The listing builds one solid part. Answer for the finished solid, in the listing's coordinates (mm). A direction names the side the tool comes from. Round coordinates to 2 decimals unless told otherwise and drop trailing zeros. Write each loop counter-clockwise with the first axis right and the second up, starting at its lowest first coordinate (ties: lowest second). Pieces come first, ordered by that corner, then holes. Notation, with made-up numbers: (31, 29) - (49, 29) arc R23 cw to (49, 66) - close; hole circle Ø8 at (25, 39). An arc over 180 degrees is marked (long way). Answer as CSV lines item,"result". Start each with the question number.
Item 1: A cutting plane is placed at A-A on y = -20.5. Determine the outline of the cut face in (x, z).
Item 2: Which of the six approach directions +Z, -Z, +X, -X, +Y, -Y give full straight-line access (tool end or side, diameter ignored) to faces 4 (the flat face through (5.197, 21, -1)), 5 (the flat face through (-21.197, -41, -1)), 6 (the flat face through (-21.197, 21, -1)), 7 (the flat face through (-13, -30.6, -1))?
Item 3: A cutting plane is placed at B-B on y = 14.65. Determine the outline of the cut face in (x, z), and give its area (3 significant figures).
Item 4: For a pull along Y with two mould halves and no side action, classify faces 1 (the flat face through (2.697, -10, -1)), 2 (the flat face through (5.197, -41, -1)), 3 (the flat face through (24, -40.1, -1)) as pulls with the +Y half, pulls with the -Y half, needs draft (parallel to the pull), parting line crosses it, or undercut.
Item 5: A flat-ended cylindrical pin translates along its axis: pin 1 (0.8 mm diameter, centred on y = -41.5, z = -1.5, fed in from +X). Find the tip coordinate at first contact, or state that the pin passes through.
Item 6: Straight lines are drawn through the part: line 1 along X through (y, z) = (-18, -0.75); line 2 along Y through (x, z) = (8, -0.4); line 3 along Y through (x, z) = (-12, -0.6). For each, find the intervals that lie inside material, in ascending order. Write a range as [from, to].
Item 7: A cutting plane is placed at D-D on z = -1.25. State how many separate pieces and enclosed holes the cut face has, and give its area (3 significant figures).
Item 8: A cutting plane is placed at C-C on x = -4. Determine the outline of the cut face in (y, z).
```python
from build123d import *

# Parameters (mm, degrees)
SKETCH_1_W      = 54
SKETCH_1_H      = 60
SKETCH_1_R      = 1.75
SKETCH_1_W_2    = 21
SKETCH_1_H_2    = 41
SKETCH_1_W_3    = 16
SKETCH_1_H_3    = 2.5
EXTRUDE_1_DEPTH = 3


with BuildPart() as part:
    # Эскиз1 → Бобышка-Вытянуть1 (new body)
    with BuildSketch(Plane.XY):
        with Locations((0, -10.1)):
            Rectangle(SKETCH_1_W, SKETCH_1_H)
        with Locations((-18.19729, 14.65)):
            Circle(SKETCH_1_R, mode=Mode.SUBTRACT)
        with Locations((-8.19729, 14.65)):
            Circle(SKETCH_1_R, mode=Mode.SUBTRACT)
        with Locations((8.19729, 14.65)):
            Circle(SKETCH_1_R, mode=Mode.SUBTRACT)
        with Locations((18.19729, 14.65)):
            Circle(SKETCH_1_R, mode=Mode.SUBTRACT)
        with Locations((18.19729, -34.85)):
            Circle(SKETCH_1_R, mode=Mode.SUBTRACT)
        with Locations((8.19729, -34.85)):
            Circle(SKETCH_1_R, mode=Mode.SUBTRACT)
        with Locations((-8.197262, -34.85)):
            Circle(SKETCH_1_R, mode=Mode.SUBTRACT)
        with Locations((-18.19729, -34.85)):
            Circle(SKETCH_1_R, mode=Mode.SUBTRACT)
        with Locations((-13.19729, -10.1)):
            Rectangle(SKETCH_1_W_2, SKETCH_1_H_2, mode=Mode.SUBTRACT)
        with Locations((13.19729, -10.1)):
            Rectangle(SKETCH_1_W_2, SKETCH_1_H_2, mode=Mode.SUBTRACT)
        with Locations((-13.19729, 21.15)):
            Rectangle(SKETCH_1_W_3, SKETCH_1_H_3)
        with Locations((13.19729, 21.15)):
            Rectangle(SKETCH_1_W_3, SKETCH_1_H_3)
        with Locations((13.19729, -41.35)):
            Rectangle(SKETCH_1_W_3, SKETCH_1_H_3)
        with Locations((-13.19729, -41.35)):
            Rectangle(SKETCH_1_W_3, SKETCH_1_H_3)
    extrude(amount=-EXTRUDE_1_DEPTH)


solid = part.part
```
Geometry says:
1,outline,"(-27, -3) - (-23.7, -3) - (-23.7, 0) - (-27, 0) - close; (-2.7, -3) - (2.7, -3) - (2.7, 0) - (-2.7, 0) - close; (23.7, -3) - (27, -3) - (27, 0) - (23.7, 0) - close"
2,face 4,"+Z, -Z, +Y"
2,face 5,"+Z, -Z, -X, -Y"
2,face 6,"+Z, -Z, -X, +Y"
2,face 7,"+Z, -Z"
3,outline,"(-27, -3) - (-19.95, -3) - (-19.95, 0) - (-27, 0) - close; (-16.45, -3) - (-9.95, -3) - (-9.95, 0) - (-16.45, 0) - close; (-6.45, -3) - (6.45, -3) - (6.45, 0) - (-6.45, 0) - close; (9.95, -3) - (16.45, -3) - (16.45, 0) - (9.95, 0) - close; (19.95, -3) - (27, -3) - (27, 0) - (19.95, 0) - close"
3,area,"120 mm^2"
4,face 1,"undercut"
4,face 2,"needs draft"
4,face 3,"pulls with the -Y half"
5,pin 1,"stops at x = 21.2"
6,line 1,"x = [-27, -23.7], [-2.7, 2.7], [23.7, 27]"
6,line 2,"y = [-42.6, -36.59], [-33.11, -30.6], [10.4, 12.91], [16.39, 22.4]"
6,line 3,"y = [-42.6, -30.6], [10.4, 22.4]"
7,separate pieces,"1"
7,enclosed holes,"10"
7,area,"1,600 mm^2"
8,outline,"(-40.1, -3) - (-30.6, -3) - (-30.6, 0) - (-40.1, 0) - close; (10.4, -3) - (19.9, -3) - (19.9, 0) - (10.4, 0) - close"
